Part model, mm, in its own coordinate system. A direction names the side the tool comes from. Round coordinates to 2 decimals unless told otherwise and drop trailing zeros. Order: outer loops, then holes, each group sorted by start corner. A loop starts at its lowest first (then second) coordinate and runs counter-clockwise, first axis right, second up. Notation, with made-up numbers: (78, 31.5) - (108, 31.5) arc R27 ccw to (108, 66.5) - close; hole circle Ø4 at (38, 20.5). An arc over 180 degrees is marked (long way). Answer as a JSON object with one key per item and string values.
Solid Edge part; units mm, degrees
sketch "Sketch1" plane through (0, 0, 0) normal (0, -1, 0) x (1, 0, 0)
  line L0 (-241.66, 15.72) -> (-241.66, 209.47)
  arc A0 (-270.34, 209.47) -> (-241.66, 209.47) centre (-256, 209.47) cw
  line L1 (-270.34, 209.47) -> (-270.34, -171.53)
  arc A1 (-241.66, -171.53) -> (-270.34, -171.53) centre (-256, -171.53) cw
  line L2 (-241.66, -171.53) -> (-241.66, -22.28)
  arc A2 (-241.66, -22.28) -> (-225.94, -6.56) centre (-225.94, -22.28) cw
  line L3 (-225.94, -6.56) -> (0, -6.56)
  line L4 (225.94, -6.56) -> (0, -6.56)
  arc A3 (241.66, -22.28) -> (225.94, -6.56) centre (225.94, -22.28) ccw
  line L5 (241.66, -171.53) -> (241.66, -22.28)
  arc A4 (241.66, -171.53) -> (270.34, -171.53) centre (256, -171.53) ccw
  line L6 (270.34, 209.47) -> (270.34, -171.53)
  arc A5 (270.34, 209.47) -> (241.66, 209.47) centre (256, 209.47) ccw
  line L7 (241.66, 15.72) -> (241.66, 209.47)
  arc A6 (225.94, 0) -> (241.66, 15.72) centre (225.94, 15.72) ccw
  line L8 (0, 0) -> (225.94, 0)
  line L9 (0, 0) -> (-225.94, 0)
  arc A7 (-225.94, 0) -> (-241.66, 15.72) centre (-225.94, 15.72) cw
  line L10 (0, -7.94) -> (-225.94, -7.94)
  arc A8 (-225.94, -7.94) -> (-240.28, -22.28) centre (-225.94, -22.28) ccw
  line L11 (-240.28, -171.53) -> (-240.28, -22.28)
  arc A9 (-271.72, -171.53) -> (-240.28, -171.53) centre (-256, -171.53) ccw
  line L12 (-271.72, 209.47) -> (-271.72, -171.53)
  arc A10 (-271.72, 209.47) -> (-240.28, 209.47) centre (-256, 209.47) cw
  line L13 (-240.28, 209.47) -> (-240.28, 15.72)
  arc A11 (-240.28, 15.72) -> (-225.94, 1.38) centre (-225.94, 15.72) ccw
  line L14 (0, 1.38) -> (-225.94, 1.38)
  line L15 (0, 1.38) -> (225.94, 1.38)
  arc A12 (240.28, 15.72) -> (225.94, 1.38) centre (225.94, 15.72) cw
  line L16 (240.28, 209.47) -> (240.28, 15.72)
  arc A13 (271.72, 209.47) -> (240.28, 209.47) centre (256, 209.47) ccw
  line L17 (271.72, 209.47) -> (271.72, -171.53)
  arc A14 (271.72, -171.53) -> (240.28, -171.53) centre (256, -171.53) cw
  line L18 (240.28, -171.53) -> (240.28, -22.28)
  arc A15 (225.94, -7.94) -> (240.28, -22.28) centre (225.94, -22.28) cw
  line L19 (0, -7.94) -> (225.94, -7.94)
extrude "Protrusion1" add sketch "Sketch1" against normal blind 6
Item 1: Two-plate mould, pull along Z, no slides. Class faces 4 (the cylindrical face through (-235.97, 2.96, -12.03)), 5 (the cylindrical face through (-256.315, 2.958, -185.867)), 6 (the cylindrical face through (-255.654, 2.958, 225.186)): pulls with the +Z half, pulls with the -Z half, needs draft (parallel to the pull), parting line crosses it, or undercut.
Taken from the geometry:
{"face 4": "pulls with the -Z half", "face 5": "undercut", "face 6": "pulls with the +Z half"}
Item 2: Cut at B-B (x = 256). Write the cut outline in (y, z), plus the area to 3 significant figures.
Taken from the geometry:
{"outline": "(0, -187.25) - (6, -187.25) - (6, -185.87) - (0, -185.87) - close; (0, 223.81) - (6, 223.81) - (6, 225.19) - (0, 225.19) - close", "area": "16.6 mm2"}
Item 3: Drop flat-ended pins along their axis: P1, Ø3, axis at x = -31.5, y = 4, coming from the -Z side; P2, Ø1.8, axis at x = 27.5, y = 4, coming from the +Z side. Give the stop position or say it passes through.
Taken from the geometry:
{"P1": "z = -7.94", "P2": "z = 1.38"}
Item 4: Cut at D-D (z = 7). Write the cut outline in (x, y), plus the area to 3 significant figures.
Taken from the geometry:
{"outline": "(-271.72, 0) - (-270.34, 0) - (-270.34, 6) - (-271.72, 6) - close; (-239.02, 0) - (-237.32, 0) - (-237.32, 6) - (-239.02, 6) - close; (237.32, 0) - (239.02, 0) - (239.02, 6) - (237.32, 6) - close; (270.34, 0) - (271.72, 0) - (271.72, 6) - (270.34, 6) - close", "area": "36.9 mm2"}
Item 5: Cut at C-C (z = 144). Write the cut outline in (x, y), plus the area to 3 significant figures.
Taken from the geometry:
{"outline": "(-271.72, 0) - (-270.34, 0) - (-270.34, 6) - (-271.72, 6) - close; (-241.66, 0) - (-240.28, 0) - (-240.28, 6) - (-241.66, 6) - close; (240.28, 0) - (241.66, 0) - (241.66, 6) - (240.28, 6) - close; (270.34, 0) - (271.72, 0) - (271.72, 6) - (270.34, 6) - close", "area": "33.1 mm2"}
Item 6: Probe L1, parallel to X at y = 1.65, z = 150; L2, parallel to Z at x = 186.5, y = 0.9; L3, parallel to X at y = 3.2, z = -4. List the from-to ranges inside material, lowest first. Write a range as from..to.
Taken from the geometry:
{"L1": "-271.72..-270.34, -241.66..-240.28, 240.28..241.66, 270.34..271.72", "L2": "-7.94..-6.56, 0..1.38", "L3": "-271.72..-270.34, 270.34..271.72"}
Item 7: Tool access for faces 1 (the cylindrical face through (256.315, 2.958, 223.807)), 2 (the cylindrical face through (-236.2, 3, 5.7)), 3 (the cylindrical face through (236.19, 2.96, -12.25)): list every direction of +Z, -Z, +X, -X, +Y, -Y with a clear straight run to the whole face (end or side of a thin tool).
Taken from the geometry:
{"face 1": "+Y, -Y", "face 2": "+Z, +Y, -Y", "face 3": "-Z, +Y, -Y"}
